Geometry check sheet. Reference: the model listing, model coordinates, mm. Face numbers are marked on the shaded views. A direction names the side the tool comes from. Give positions to 0.01 mm unless a question says otherwise; leave off trailing zeros. Write each loop counter-clockwise with the first axis right and the second up, starting at its lowest first coordinate (ties: lowest second). Pieces come first, ordered by that corner, then holes. Notation, with made-up numbers: (36, 20.25) - (57, 20.25) arc R28 cw to (57, 58.25) - close; hole circle Ø3 at (36, -29.75). An arc over 180 degrees is marked (long way). Write item = value, one per line. Start each with the question number.
(1) Section check A-A, the plane z = -25.4. Enter the section's corners in (x, y) (3 decimals), plus the area to 3 significant figures.
(2) Depth check by flat-ended pin: pin 1 Ø6 at (x, y) = (-1.5, 5.5) entering from -Z; pin 2 Ø2.5 at (x, y) = (5.5, 8) entering from -Z; pin 3 Ø0.6 at (x, z) = (-2.5, -25) entering from +Y. Enter the tip coordinate at first touch or a pass-through.
(3) Section check C-C, the plane z = 3.5. Enter the section's corners in (x, y) (3 decimals).
(4) Section check D-D, the plane y = 6.5. Enter the section's corners in (x, z).
(5) Thickness scan on L1, parallel to Y at x = -11, z = 14.5; L2, parallel to Z at x = 9, y = 8; L3, parallel to X at y = 4.5, z = -7. Record the ranges inside material, lowest first.
(6) Section check B-B, the plane x = -2.54. Enter the section's corners in (y, z) (3 decimals), plus the area to 3 significant figures.
(7) Draft check along X on the marked faces 1 and 2. Enter one of: pulls with the +X half, pulls with the -X half, needs draft (parallel to the pull), parting line crosses it, or undercut.
(8) Access from +Z, -Z, +X, -X, +Y, -Y to the whole of each face (thin tool, end or side, straight path). Record for the marked faces 3 and 4.
```python
from build123d import *

# Parameters (mm, degrees)
SKETCH1_W           = 34.29
SKETCH1_H           = 55.88
BOSS_EXTRUDE1_DEPTH = 4.318
SKETCH2_W           = 34.29
SKETCH2_H           = 50.8
BOSS_EXTRUDE2_DEPTH = 6.35
SKETCH3_OUTSIDE_W   = 49.574
SKETCH3_OUTSIDE_H   = 25.952
CUT_EXTRUDE1_DEPTH  = 5.08
CUT_EXTRUDE2_DEPTH  = 55.666234999
SKETCH6_R           = 0.635
CUT_EXTRUDE3_DEPTH  = 0.127


with BuildPart() as part:
    # Sketch1 → Boss-Extrude1 (new body)
    with BuildSketch(Plane(origin=(0, 0, 0), x_dir=(1, 0, 0), z_dir=(0, 1, 0))):
        Rectangle(SKETCH1_W, SKETCH1_H)
    extrude(amount=BOSS_EXTRUDE1_DEPTH)

    # Sketch2 → Boss-Extrude2 (add)
    with BuildSketch(Plane(origin=(0, 4.318, 0), x_dir=(1, 0, 0), z_dir=(0, 1, 0))):
        with Locations((0, -2.54)):
            Rectangle(SKETCH2_W, SKETCH2_H)
    extrude(amount=BOSS_EXTRUDE2_DEPTH)

    # Sketch3 outside → Cut-Extrude1 (cut)
    with BuildSketch(Plane(origin=(0, 0, -27.94), x_dir=(-1, 0, 0), z_dir=(0, 0, -1))):
        with Locations((0, 5.334)):
            Rectangle(SKETCH3_OUTSIDE_W, SKETCH3_OUTSIDE_H)
        with BuildLine():
            Line((-15.875, 0), (15.875, 0))
            ThreePointArc((15.875, 0), (16.773025612, 0.371974388), (17.145, 1.27))
            Line((17.145, 1.27), (17.145, 3.048))
            ThreePointArc((17.145, 3.048), (16.773025612, 3.946025612), (15.875, 4.318))
            Line((15.875, 4.318), (-15.875, 4.318))
            ThreePointArc((-15.875, 4.318), (-16.773025612, 3.946025612), (-17.145, 3.048))
            Line((-17.145, 3.048), (-17.145, 1.27))
            ThreePointArc((-17.145, 1.27), (-16.773025612, 0.371974388), (-15.875, 0))
        make_face(mode=Mode.SUBTRACT)
    extrude(amount=-CUT_EXTRUDE1_DEPTH, mode=Mode.SUBTRACT)

    # Sketch4 → Cut-Extrude2 (cut, through all)
    with BuildSketch(Plane(origin=(0, 0, -22.86), x_dir=(-1, 0, 0), z_dir=(0, 0, -1))):
        with BuildLine():
            Line((-17.145, 10.668), (-17.145, 4.318))
            ThreePointArc((-17.145, 4.318), (-15.285128061, 8.808128061), (-10.795, 10.668))
            Line((-10.795, 10.668), (-17.145, 10.668))
        make_face()
        with BuildLine():
            Line((17.145, 10.668), (10.795, 10.668))
            ThreePointArc((10.795, 10.668), (15.285128061, 8.808128061), (17.145, 4.318))
            Line((17.145, 4.318), (17.145, 10.668))
        make_face()
        with BuildLine():
            Line((-17.145, 1.27), (-17.145, 0))
            Line((-17.145, 0), (-15.875, 0))
            ThreePointArc((-15.875, 0), (-16.773025612, 0.371974388), (-17.145, 1.27))
        make_face()
        with BuildLine():
            Line((17.145, 0), (17.145, 1.27))
            ThreePointArc((17.145, 1.27), (16.773025612, 0.371974388), (15.875, 0))
            Line((15.875, 0), (17.145, 0))
        make_face()
    extrude(amount=-CUT_EXTRUDE2_DEPTH, mode=Mode.SUBTRACT)

    # Sketch6 → Cut-Extrude3 (cut)
    with BuildSketch(Plane(origin=(0, 4.318, 0), x_dir=(1, 0, 0), z_dir=(0, 1, 0))):
        with Locations(Location((-2.54, 25.4, 0), (0, 0, 270))):
            Circle(SKETCH6_R)
        with Locations(Location((2.54, 25.4, 0), (0, 0, 90))):
            Circle(SKETCH6_R)
    extrude(amount=-CUT_EXTRUDE3_DEPTH, mode=Mode.SUBTRACT)


solid = part.part
```
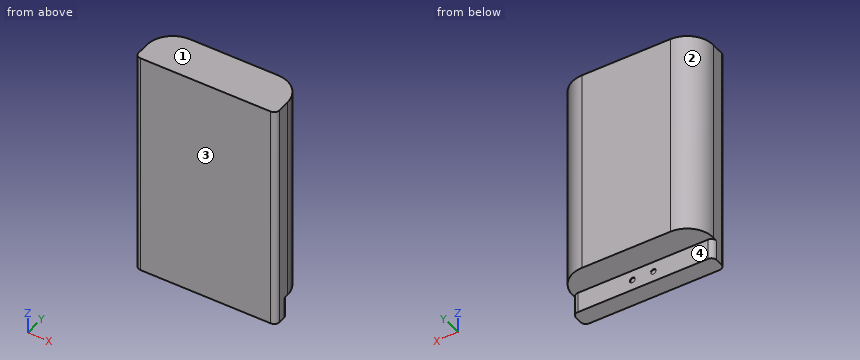
Model answer:
q1.outline = (-17.145, 1.27) arc R1.27 ccw to (-15.875, 0) - (15.875, 0) arc R1.27 ccw to (17.145, 1.27) - (17.145, 3.048) arc R1.27 ccw to (15.875, 4.318) - (3.175, 4.318) - (3.175, 4.191) - (1.905, 4.191) - (1.905, 4.318) - (-1.905, 4.318) - (-1.905, 4.191) - (-3.175, 4.191) - (-3.175, 4.318) - (-15.875, 4.318) arc R1.27 ccw to (-17.145, 3.048) - close
q1.area = 146 mm²
q2.pin_1 = -27.94
q2.pin_2 = -22.86
q2.pin_3 = 4.32
q3.outline = (-17.145, 1.27) arc R1.27 ccw to (-15.875, 0) - (15.875, 0) arc R1.27 ccw to (17.145, 1.27) - (17.145, 4.318) arc R6.35 ccw to (10.795, 10.668) - (-10.795, 10.668) arc R6.35 ccw to (-17.145, 4.318) - close
q4.outline = (-16.76, -22.86) - (16.76, -22.86) - (16.76, 27.94) - (-16.76, 27.94) - close
q5.L1 = 0 to 10.66
q5.L2 = -22.86 to 27.94
q5.L3 = -17.14 to 17.14
q6.outline = (0, -27.94) - (4.318, -27.94) - (4.318, -26.035) - (4.191, -26.035) - (4.191, -24.765) - (4.318, -24.765) - (4.318, -22.86) - (10.668, -22.86) - (10.668, 27.94) - (0, 27.94) - close
q6.area = 564 mm²
q7.face_1 = needs draft
q7.face_2 = pulls with the -X half
q8.face_3 = +Z, -Z, +X, -X, -Y
q8.face_4 = -Z, +X, -X, +Y
